Check sheet for the modelled part. Datum: model origin and axes. Units: mm. Face numbers are marked on the shaded views. A direction names the side the tool comes from. Give positions to 0.01 mm unless a question says otherwise; leave off trailing zeros. Write each loop counter-clockwise with the first axis right and the second up, starting at its lowest first coordinate (ties: lowest second). Pieces come first, ordered by that corner, then holes. Notation, with made-up numbers: (-30, 24.5) -> (14, 24.5) arc R9 ccw to (14, 28.5) -> close; hole circle Ø9 at (-16, 15.5). An arc over 180 degrees is marked (long way). Use a Markdown table: item, result. Add a question column.
1. Cross-section at D-D (z = -12.25). Enter the section's corners in (x, y).
2. Set-up check for the marked faces 1 and 2: record each of +Z, -Z, +X, -X, +Y, -Y from which the full face is reachable in a straight line by a thin tool's end or side.
3. Cross-section at B-B (y = 4). Enter the section's corners in (x, z).
4. Cross-section at A-A (x = 2.1). Enter the section's corners in (y, z).
5. Scan lines: probe 1 along Y at (x, z) = (0.75, -13.5); probe 2 along X at (y, z) = (1.3, -10); probe 3 along Z at (x, y) = (2.1, 1.7). Record each from-to range of solid material in increasing order. Write a range as [from, to].
6. Cross-section at C-C (x = 0). Enter the section's corners in (y, z), then the cut area to 3 significant figures.
7. Gauge pin test, flat ends, axial feed: P1, Ø3, axis at x = 1, z = -10, coming from the +Y side; P2, Ø1.3, axis at x = 2.1, z = -10, coming from the -Y side. Record the tip position at first contact, or that the pin passes through.
from build123d import *

# Parameters (mm, degrees)
F1_DEPTH = 14
F2_W     = 6.2
F2_H     = 8.5
F3_DEPTH = 14
F6_D     = 2.1
F7_R     = 1.5


with BuildPart() as f1:
    # F0 (on Front) → F1 (new body)
    with BuildSketch(Plane.XZ):
        with BuildLine():
            Line((3.1, -20), (3.1, 0))
            ThreePointArc((3.1, 0), (0, 3.1), (-3.1, 0))
            Line((-3.1, 0), (-3.1, -20))
            Line((-3.1, -20), (3.1, -20))
        make_face()
    extrude(amount=-F1_DEPTH)

    # F2 (on face) → F3 (cut)
    with BuildSketch(Plane(origin=(0, 0, -20), x_dir=(1, 0, 0), z_dir=(0, 0, -1))):
        with Locations((0, -9.75)):
            Rectangle(F2_W, F2_H)
    extrude(amount=-F3_DEPTH, mode=Mode.SUBTRACT)

    # F6 (through all)
    with Locations(Plane.XZ.offset(5)):
        with Locations((2.1, -10)):
            Hole(F6_D / 2)

    # F7
    f7_edges = [f1.edges().sort_by_distance(p)[0] for p in [
        (3.1, 2.75, -20),
        (-3.1, 2.75, -20),
    ]]
    fillet(f7_edges, radius=F7_R)


solid = f1.part
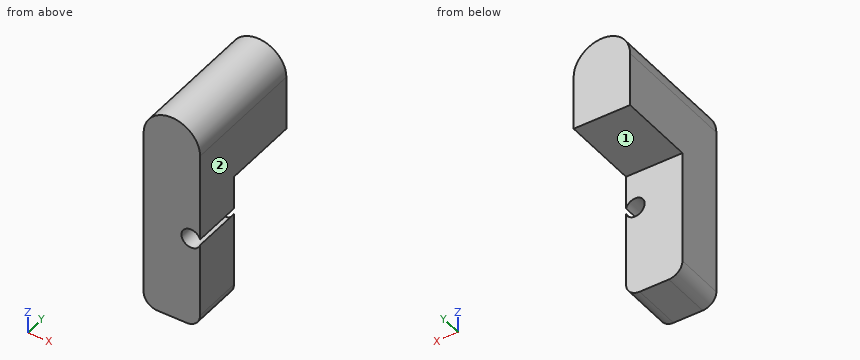
Worked answers:
| question | item | result |
|---|---|---|
| 1 | outline | (-3.1, 0) -> (3.1, 0) -> (3.1, 5.5) -> (-3.1, 5.5) -> close |
| 2 | face 1 | -Z, +X, -X, +Y |
| 2 | face 2 | +Z, -Z, +X, +Y, -Y |
| 3 | outline | (-3.1, -18.5) arc R1.5 ccw to (-1.6, -20) -> (1.6, -20) arc R1.5 ccw to (3.1, -18.5) -> (3.1, -10.32) arc R1.05 cw (long way) to (3.1, -9.68) -> (3.1, 0) arc R3.1 ccw to (-3.1, 0) -> close |
| 4 | outline | (0, -19.91) -> (5.5, -19.91) -> (5.5, -11.05) -> (0, -11.05) -> close; (0, -8.95) -> (5.5, -8.95) -> (5.5, -6) -> (14, -6) -> (14, 2.28) -> (0, 2.28) -> close |
| 5 | probe 1 | y = [0, 5.5] |
| 5 | probe 2 | x = [-3.1, 1.05] |
| 5 | probe 3 | z = [-19.91, -11.05], [-8.95, 2.28] |
| 6 | outline | (0, -20) -> (5.5, -20) -> (5.5, -6) -> (14, -6) -> (14, 3.1) -> (0, 3.1) -> close |
| 6 | area | 204 mm² |
| 7 | P1 | stops at y = 5.5 |
| 7 | P2 | passes through |
